```python
from build123d import *

# Parameters (mm, degrees)
F0_R     = 7.5
F0_R_2   = 43.5
F1_DEPTH = 90


with BuildPart() as f1:
    # F0 (on Front) → F1 (new body)
    with BuildSketch(Plane.XZ):
        with BuildLine():
            Line((-59.710717, -38.00515), (-45.230323, -33.356527))
            ThreePointArc((-45.230323, -33.356527), (-0.022679, -56.199995), (45.203387, -33.39302))
            Line((45.203387, -33.39302), (61.163897, -38.509449))
            ThreePointArc((61.163897, -38.509449), (83.799497, -26.863437), (72.153485, -4.227837))
            Line((72.153485, -4.227837), (56.192975, 0.888592))
            ThreePointArc((56.192975, 0.888592), (45.401571, 33.123063), (18, 53.239459))
            Line((18, 53.239459), (18, 69.999847))
            ThreePointArc((18, 69.999847), (0, 87.999847), (-18, 69.999847))
            Line((-18, 69.999847), (-18, 53.239459))
            ThreePointArc((-18, 53.239459), (-45.408469, 33.113607), (-56.19334, 0.865185))
            Line((-56.19334, 0.865185), (-72.151649, -4.25789))
            ThreePointArc((-72.151649, -4.25789), (-83.538616, -27.622503), (-59.710717, -38.00515))
        make_face()
        with Locations((-66.649695, -21.3964)):
            Circle(F0_R, mode=Mode.SUBTRACT)
        Circle(F0_R_2, mode=Mode.SUBTRACT)
        with Locations((66.658691, -21.368643)):
            Circle(F0_R, mode=Mode.SUBTRACT)
        with Locations((0, 69.999847)):
            Circle(F0_R, mode=Mode.SUBTRACT)
    extrude(amount=F1_DEPTH)


solid = f1.part
```
Part model, mm, in its own coordinate system. A direction names the side the tool comes from. Round coordinates to 2 decimals unless told otherwise and drop trailing zeros. Loops run counter-clockwise (first coordinate to the right, second up) from the corner with the lowest first, then second, coordinate; pieces in that order, holes last.
1. Slice it at C-C (y = -50.5). Give the cut face in (x, z), and give its area (3 significant figures).
Solutions:
outline: (-72.15, -4.26) arc R18 ccw (long way) to (-59.71, -38.01) - (-45.23, -33.36) arc R56.2 ccw to (45.2, -33.39) - (61.16, -38.51) arc R18 ccw to (72.15, -4.23) - (56.19, 0.89) arc R56.2 ccw to (18, 53.24) - (18, 70) arc R18 ccw to (-18, 70) - (-18, 53.24) arc R56.2 ccw to (-56.19, 0.87) - close; hole circle Ø15 at (-66.65, -21.4); hole circle Ø87 at (0, 0); hole circle Ø15 at (0, 70); hole circle Ø15 at (66.66, -21.37)
area: 6,570 mm2
2. Two-plate mould, pull along X, no slides. Class faces 1 (the face through (-18, -44, 62)), 2 (the face through (-74.142, -44.37, -21.067)), 3 (the face through (18, -44, 62)), 4 (the face through (0, -44, 88)): pulls with the +X half, pulls with the -X half, needs draft (parallel to the pull), parting line crosses it, or undercut.
Solutions:
face 1: pulls with the -X half
face 2: undercut
face 3: pulls with the +X half
face 4: parting line crosses it
3. 3-axis set-ups, long thin cutter, end or side, ignore diameter. For faces 5 (the face through (-52.572, -44.37, -35.713)), 6 (the face through (-44, 0, 0)): which of +Z, -Z, +X, -X, +Y, -Y reach the whole face in a straight line?
Solutions:
face 5: -Z, +Y, -Y
face 6: +Z, -Z, +X, -X, +Y
4. Slice it at D-D (x = -62). Give the cut face in (y, z), and give its area (3 significant figures).
Solutions:
outline: (-90, -38.79) - (0, -38.79) - (0, -27.28) - (-90, -27.28) - close; (-90, -15.51) - (0, -15.51) - (0, -1) - (-90, -1) - close
area: 2,340 mm2
5. Slice it at A-A (x = 0). Give the cut face in (y, z).
Solutions:
outline: (-90, -56.2) - (0, -56.2) - (0, -43.5) - (-90, -43.5) - close; (-90, 43.5) - (0, 43.5) - (0, 62.5) - (-90, 62.5) - close; (-90, 77.5) - (0, 77.5) - (0, 88) - (-90, 88) - close
6. Slice it at B-B (z = 32). Give the cut face in (x, y).
Solutions:
outline: (-46.2, -90) - (-29.47, -90) - (-29.47, 0) - (-46.2, 0) - close; (29.47, -90) - (46.2, -90) - (46.2, 0) - (29.47, 0) - close
7. Flat gauge pins, fed straight in: pin 1 (8 mm diameter, centred on x = -2.5, y = -55, fed in from -Z); pin 2 (4 mm diameter, centred on x = -65.5, y = -60, fed in from +Z); pin 3 (1 mm diameter, centred on x = -19.5, y = -55.5, fed in from -Z). Where does each tip first touch, or does it go through?
Solutions:
pin 1: stops at z = -56.2
pin 2: stops at z = -1.48
pin 3: stops at z = -52.89
8. Drill centre lines: line 1 along Z through (x, y) = (0, -63); line 2 along X through (y, z) = (-11, -26.5); line 3 along X through (y, z) = (-77.5, -25). Where is each one in solid material? Low to high.
Solutions:
line 1: z = -56.2 to -43.5, 43.5 to 62.5, 77.5 to 88
line 2: x = -83.91 to -72.15, -61.15 to -34.5, 34.5 to 61.19, 72.13 to 83.91
line 3: x = -84.29 to -73.23, -60.07 to -35.6, 35.6 to 60.1, 73.22 to 84.29
